Source: three-view drawing plus pictorial views. Frame: mm from the lowest corner of the part. A direction names the side the tool comes from. Give positions to 0.01 mm unless a question says otherwise; leave off trailing zeros. Write each loop counter-clockwise with the first axis right and the second up, starting at its lowest first coordinate (ties: lowest second). Pieces come first, ordered by that corner, then holes. Notation, with made-up numbers: M 8,-14 L 60,-14 A20 ccw 60,18 Z; hole C 11.5,68 d11. An arc over 180 degrees is marked long. Return JSON: item names as keys, results as strings.
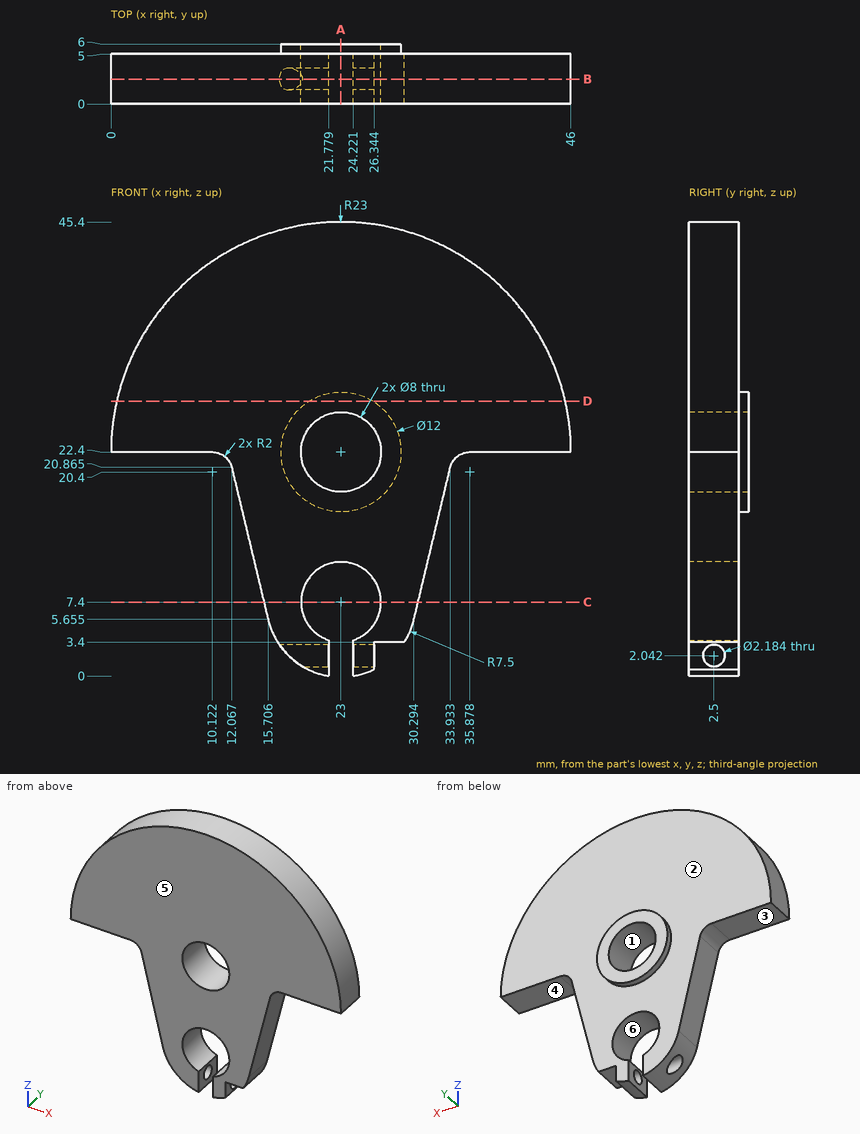
1) Line query: line 1 (Z direction, x = 26, y = 3) (1 decimal); line 2 (Z direction, x = 26, y = 0.75) (1 decimal); line 3 (Y direction, x = 17.5, z = 30.5). Output: solid intervals per line, ascending. Write a range as [from, to].
Numbers:
{"line 1": "z = [0.5, 1.1], [3, 4.8], [10, 19.8], [25, 45.2]", "line 2": "z = [0.5, 4.8], [10, 19.8], [25, 45.2]", "line 3": "y = [0, 5]"}
2) Cut plane D-D, the plane z = 27.5. Return the cut outline in (x, y).
Numbers:
{"outline": "M 0.57,0 L 45.43,0 L 45.43,5 L 26.16,5 L 26.16,6 L 19.84,6 L 19.84,5 L 0.57,5 Z"}
3) Draft query along Z for the marked faces 4, 5 and 6. Return one class per face: released by +Z, released by -Z, zero draft, split by the parting line, or undercut.
Numbers:
{"face 4": "released by -Z", "face 5": "zero draft", "face 6": "undercut"}
4) Cut plane A-A, the plane x = 23. Return the cut outline in (y, z).
Numbers:
{"outline": "M 0,11.4 L 5,11.4 L 5,16.4 L 6,16.4 L 6,18.4 L 0,18.4 Z; M 0,26.4 L 6,26.4 L 6,28.4 L 5,28.4 L 5,45.4 L 0,45.4 Z"}
5) Cut plane C-C, the plane z = 7.4. Return the cut outline in (x, y), then the cut area to 3 significant figures.
Numbers:
{"outline": "M 15.29,0 L 19,0 L 19,5 L 15.29,5 Z; M 27,0 L 30.71,0 L 30.71,5 L 27,5 Z", "area": "37.1 mm²"}
6) Contact query for flat-ended pins moving along their axis: pin 1 Ø3 at (y, z) = (2, 2.5) entering from +X (1 decimal); pin 2 Ø2.5 at (x, y) = (27, 3) entering from -Z; pin 3 Ø2 at (y, z) = (2, 2.5) entering from +X. Output: stop coordinate, or through.
Numbers:
{"pin 1": "stops at x = 29.7", "pin 2": "stops at z = 0.42", "pin 3": "stops at x = 29.41"}
7) Cut plane B-B, the plane y = 2.5. Give the number of separate pieces and of enclosed holes in the cut face, then the cut area to 3 significant figures.
Numbers:
{"separate pieces": "3", "enclosed holes": "1", "area": "1,080 mm²"}
8) Set-up query: the marked faces 1, 2 and 3. Return all of +Z, -Z, +X, -X, +Y, -Y with unobstructed straight access to the full face (end or side cutting, diameter ignored); none if empty.
Numbers:
{"face 1": "+Y, -Y", "face 2": "+Y", "face 3": "-Z, -X, +Y, -Y"}
